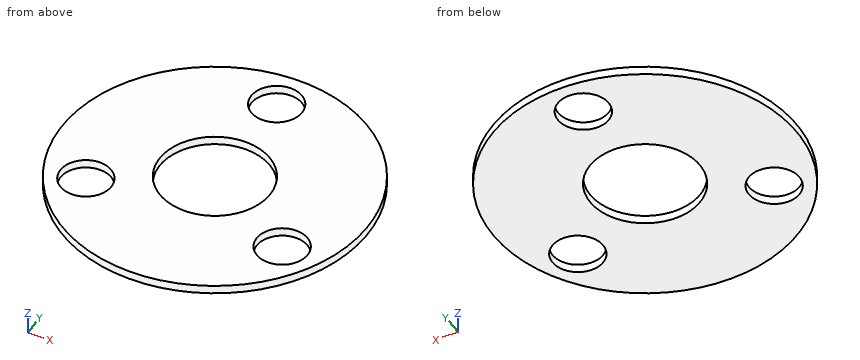
from build123d import *

# Parameters (mm, degrees)
CROQUIS1_R              = 18
SALIENTE_EXTRUIR2_DEPTH = 1
CROQUIS5_R              = 3
CROQUIS5_R_2            = 6.5
CORTAR_EXTRUIR3_DEPTH   = 1


with BuildPart() as part:
    # Croquis1 → Saliente-Extruir2 (new body)
    with BuildSketch(Plane.XY):
        Circle(CROQUIS1_R)
    extrude(amount=SALIENTE_EXTRUIR2_DEPTH)

    # Croquis5 → Cortar-Extruir3 (cut)
    with BuildSketch(Plane.XY.offset(1)):
        with Locations((0, 13.5)):
            Circle(CROQUIS5_R)
        with Locations((11.691342951, -6.75)):
            Circle(CROQUIS5_R)
        with Locations((-11.691342951, -6.75)):
            Circle(CROQUIS5_R)
        Circle(CROQUIS5_R_2)
    extrude(amount=-CORTAR_EXTRUIR3_DEPTH, mode=Mode.SUBTRACT)


solid = part.part
Part model, mm, in its own coordinate system. Give positions to 0.01 mm unless a question says otherwise; leave off trailing zeros. Loops run counter-clockwise (first coordinate to the right, second up) from the corner with the lowest first, then second, coordinate; pieces in that order, holes last.
(1) Drill centre lines: line 1 along Y through (x, z) = (0, 0.75); line 2 along Y through (x, z) = (2, 0.65); line 3 along X through (y, z) = (11.5, 0.15). Where is each one in solid material? Low to high.
Return value:
line 1: y = -18 to -6.5, 6.5 to 10.5, 16.5 to 18
line 2: y = -17.89 to -6.18, 6.18 to 11.26, 15.74 to 17.89
line 3: x = -13.85 to -2.24, 2.24 to 13.85
(2) Band-saw the part on C-C (z = 0.8). Write the cut outline in (x, y), and give its area (3 significant figures).
Return value:
outline: circle Ø36 at (0, 0); hole circle Ø6 at (-11.69, -6.75); hole circle Ø13 at (0, 0); hole circle Ø6 at (0, 13.5); hole circle Ø6 at (11.69, -6.75)
area: 800 mm2
(3) Band-saw the part on A-A (y = 0). Write the cut outline in (x, z).
Return value:
outline: (-18, 0) - (-6.5, 0) - (-6.5, 1) - (-18, 1) - close; (6.5, 0) - (18, 0) - (18, 1) - (6.5, 1) - close
(4) Band-saw the part on B-B (x = 0). Write the cut outline in (y, z), and give its area (3 significant figures).
Return value:
outline: (-18, 0) - (-6.5, 0) - (-6.5, 1) - (-18, 1) - close; (6.5, 0) - (10.5, 0) - (10.5, 1) - (6.5, 1) - close; (16.5, 0) - (18, 0) - (18, 1) - (16.5, 1) - close
area: 17.0 mm2
(5) Band-saw the part on D-D (x = -4.5). Write the cut outline in (y, z), and give its area (3 significant figures).
Return value:
outline: (-17.43, 0) - (-4.69, 0) - (-4.69, 1) - (-17.43, 1) - close; (4.69, 0) - (17.43, 0) - (17.43, 1) - (4.69, 1) - close
area: 25.5 mm2
